Read the model definition and answer for the solid it produces. Units are mm, in the model's axes. Face numbers are marked on the shaded views. A direction names the side the tool comes from. Round coordinates to 2 decimals unless told otherwise and drop trailing zeros. Order: outer loops, then holes, each group sorted by start corner. A loop starts at its lowest first (then second) coordinate and runs counter-clockwise, first axis right, second up.
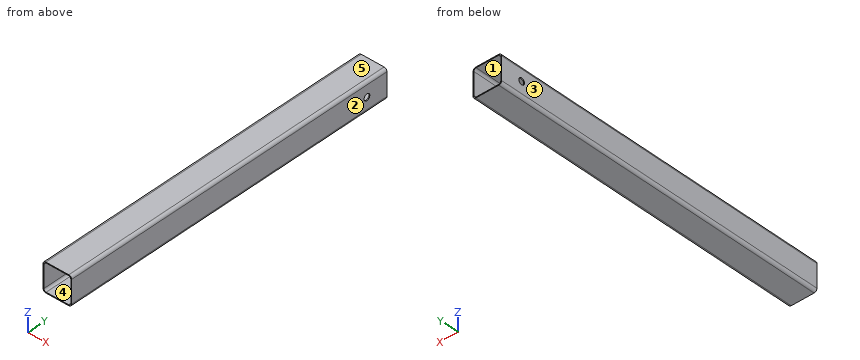
from build123d import *

# Parameters (mm, degrees)
F1_DEPTH = 600
F2_R     = 5.5
F3_DEPTH = 100


with BuildPart() as f1:
    # F0 (on Front) → F1 (new body)
    with BuildSketch(Plane.XZ):
        with BuildLine():
            ThreePointArc((2.020508, 5), (3.484974, 1.464466), (7.020508, 0))
            Line((7.020508, 0), (47.020508, 0))
            ThreePointArc((47.020508, 0), (50.556042, 1.464466), (52.020508, 5))
            Line((52.020508, 5), (52.020508, 45))
            ThreePointArc((52.020508, 45), (50.556042, 48.535534), (47.020508, 50))
            Line((47.020508, 50), (7.020508, 50))
            ThreePointArc((7.020508, 50), (3.484974, 48.535534), (2.020508, 45))
            Line((2.020508, 45), (2.020508, 5))
        make_face()
        with BuildLine():
            ThreePointArc((7.520508, 1.5), (4.692081, 2.671573), (3.520508, 5.5))
            Line((3.520508, 5.5), (3.520508, 44.5))
            ThreePointArc((3.520508, 44.5), (4.692081, 47.328427), (7.520508, 48.5))
            Line((7.520508, 48.5), (46.520508, 48.5))
            ThreePointArc((46.520508, 48.5), (49.348935, 47.328427), (50.520508, 44.5))
            Line((50.520508, 44.5), (50.520508, 5.5))
            ThreePointArc((50.520508, 5.5), (49.348935, 2.671573), (46.520508, 1.5))
            Line((46.520508, 1.5), (7.520508, 1.5))
        make_face(mode=Mode.SUBTRACT)
    extrude(amount=F1_DEPTH)

    # F2 (on face) → F3 (cut)
    with BuildSketch(Plane.YZ.offset(52.020508)):
        with Locations((-38.1458, 25)):
            Circle(F2_R)
    extrude(amount=-F3_DEPTH, mode=Mode.SUBTRACT)


solid = f1.part
Q1. For the marked faces 1 and 2, determine the directions among +Z, -Z, +X, -X, +Y, -Y from which every point of the face is accessible in a straight line to the end or side of a thin tool.
Outcome:
face 1: +Y, -Y
face 2: +Z, -Z, +X, +Y, -Y
Q2. A cutting plane is placed at C-C, the plane x = 34. Give the vertices of the cut face in (y, z), plus the area to 3 significant figures.
Outcome:
outline: (-600, 0) - (0, 0) - (0, 1.5) - (-600, 1.5) - close; (-600, 48.5) - (0, 48.5) - (0, 50) - (-600, 50) - close
area: 1,800 mm2
Q3. A cutting plane is placed at B-B, the plane y = -66. Give the vertices of the cut face in (x, z), plus the area to 3 significant figures.
Outcome:
outline: (2.02, 5) arc R5 ccw to (7.02, 0) - (47.02, 0) arc R5 ccw to (52.02, 5) - (52.02, 45) arc R5 ccw to (47.02, 50) - (7.02, 50) arc R5 ccw to (2.02, 45) - close; hole (3.52, 5.5) arc R4 ccw to (7.52, 1.5) - (46.52, 1.5) arc R4 ccw to (50.52, 5.5) - (50.52, 44.5) arc R4 ccw to (46.52, 48.5) - (7.52, 48.5) arc R4 ccw to (3.52, 44.5) - close
area: 283 mm2
Q4. For a pull along X with two mould halves and no side action, classify the marked faces 3, 4 and 5 as released by +X, released by -X, zero draft, split by the parting line, or undercut.
Outcome:
face 3: released by -X
face 4: undercut
face 5: zero draft
Q5. A cutting plane is placed at A-A, the plane z = 25. Give the vertices of the cut face in (x, y), plus the area to 3 significant figures.
Outcome:
outline: (2.02, -600) - (3.52, -600) - (3.52, -43.65) - (2.02, -43.65) - close; (2.02, -32.65) - (3.52, -32.65) - (3.52, 0) - (2.02, 0) - close; (50.52, -600) - (52.02, -600) - (52.02, -43.65) - (50.52, -43.65) - close; (50.52, -32.65) - (52.02, -32.65) - (52.02, 0) - (50.52, 0) - close
area: 1,770 mm2
Q6. Straight lines are drawn through the part: probe 1 along X at (y, z) = (-538, 39.5); probe 2 along X at (y, z) = (-544, 5); probe 3 along Z at (x, y) = (32, -349). For each, find the intervals that lie inside material, in ascending order.
Outcome:
probe 1: x = 2.02 to 3.52, 50.52 to 52.02
probe 2: x = 2.02 to 3.55, 50.49 to 52.02
probe 3: z = 0 to 1.5, 48.5 to 50
Q7. A flat-ended cylindrical pin translates along its axis: pin 1 (12.5 mm diameter, centred on y = -38.15, z = 25, fed in from -X). Find the tip coordinate at first contact, or state that the pin passes through.
Outcome:
pin 1: stops at x = 2.02
